from build123d import *

# Parameters (mm, degrees)
F0_R     = 50.157501
F1_DEPTH = 10
F2_R     = 3.626246
F4_R     = 6
F5_DEPTH = 25
F6_R     = 3.797047
F7_DEPTH = 100


with BuildPart() as f1:
    # F0 (on Front) → F1 (new body)
    with BuildSketch(Plane.XZ):
        Circle(F0_R)
    extrude(amount=-F1_DEPTH)

    # F2 (on Right) → F3 (revolve, cut)
    with BuildSketch(Plane.YZ):
        with Locations((5.051546, 50.064437)):
            Circle(F2_R)
    revolve(axis=Axis((0, -2.255155, 0), (0, 1, 0)), mode=Mode.SUBTRACT)

    # F4 (on face) → F5 (join)
    with BuildSketch(Plane.XZ):
        Circle(F4_R)
    extrude(amount=F5_DEPTH)


with BuildPart() as f7:
    # F6 (on Right) → F7 (new body, symmetric)
    with BuildSketch(Plane.YZ):
        with Locations((0, 74.842192)):
            Circle(F6_R)
    extrude(amount=F7_DEPTH, both=True)


solid = f1.part
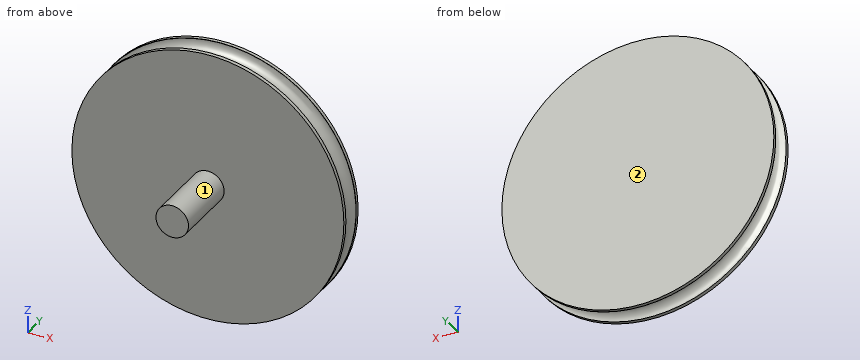
Input: part model. Units: mm. Frame: model coordinates. Face numbers are marked on the shaded views. A direction names the side the tool comes from. Give positions to 0.01 mm unless a question says otherwise; leave off trailing zeros. Write each loop counter-clockwise with the first axis right and the second up, starting at its lowest first coordinate (ties: lowest second). Pieces come first, ordered by that corner, then holes. Notation, with made-up numbers: M 62,3 L 68,3 A19 ccw 68,9 Z; hole C 1,80 d1. An arc over 180 degrees is marked long. Use one line per item in the form item = value.
1. Cut plane B-B on x = 0. Return loops of the section in (y, z), and give its area (3 significant figures).
Outcome:
outline = M -25,-6 L 0,-6 L 0,-50.16 L 1.43,-50.16 A3.63 cw long 8.68,-50.16 L 10,-50.16 L 10,50.16 L 8.68,50.16 A3.63 cw long 1.43,50.16 L 0,50.16 L 0,6 L -25,6 Z
area = 1,260 mm²
2. Reachability of the marked faces 1 and 2 from +Z, -Z, +X, -X, +Y, -Y: full face, straight path, thin tool, end or side. Return the list, or none.
Outcome:
face_1 = -Y
face_2 = +Z, -Z, +X, -X, +Y
3. Cut plane C-C on y = -2. Return loops of the section in (x, z), and give its area (3 significant figures).
Outcome:
outline = C 0,0 d12
area = 113 mm²
4. Cut plane A-A on z = 0. Return loops of the section in (x, y).
Outcome:
outline = M -50.16,0 L -6,0 L -6,-25 L 6,-25 L 6,0 L 50.16,0 L 50.16,1.43 A3.63 cw long 50.16,8.68 L 50.16,10 L -50.16,10 L -50.16,8.68 A3.63 cw long -50.16,1.43 Z
5. Ray query, L1, parallel to Y at x = 10.5, z = -30; L2, parallel to X at y = -22.5, z = 0.5; L3, parallel to Z at x = 26, y = 3.5. Return the intervals inside material, ascending.
Outcome:
L1 = 0 to 10
L2 = -5.98 to 5.98
L3 = -38.9 to 38.9
6. First-contact query: P1, Ø2, axis at y = 5.5, z = 3.5, coming from the -X side; P2, Ø12, axis at x = -7, z = 27.5, coming from the -Y side; P3, Ø5, axis at x = -1, y = 5.5, coming from the -Z side. Flat tips, straight axial feed; report the tip coordinate or a pass-through.
Outcome:
P1 = -46.61
P2 = 0
P3 = -47.94
